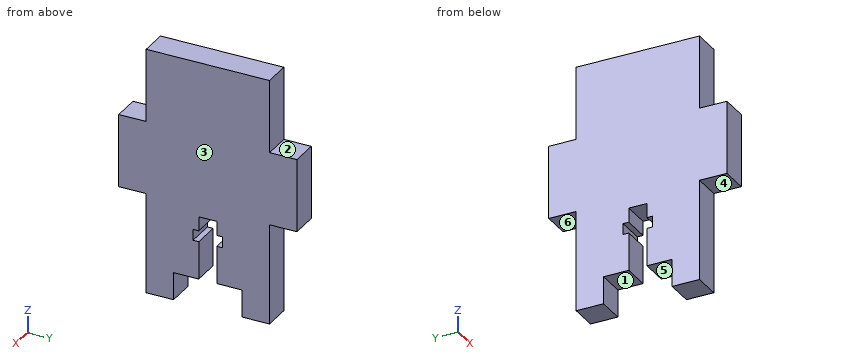
from build123d import *

# Parameters (mm, degrees)
SKETCH1_W           = 6.35
SKETCH1_H           = 28.575
BOSS_EXTRUDE1_DEPTH = 50.8
BOSS_EXTRUDE2_START = -34.925
SKETCH2_W           = 6.35
SKETCH2_H           = 16.933333334
BOSS_EXTRUDE2_DEPTH = 41.275
SKETCH3_W           = 6.35
SKETCH3_H           = 6.35
BOSS_EXTRUDE3_DEPTH = 6.35
CUT_EXTRUDE1_DEPTH  = 56.198450216


with BuildPart() as part:
    # Sketch1 → Boss-Extrude1 (new body)
    with BuildSketch(Plane.XY):
        with Locations((-25.4, 0)):
            Rectangle(SKETCH1_W, SKETCH1_H)
    extrude(amount=BOSS_EXTRUDE1_DEPTH)

    # Sketch2 → Boss-Extrude2 (add)
    with BuildSketch(Plane(origin=(0, -14.2875, 0), x_dir=(-1, 0, 0), z_dir=(0, -1, 0)).offset(BOSS_EXTRUDE2_START)):
        with Locations((25.4, -25.4)):
            Rectangle(SKETCH2_W, SKETCH2_H)
    extrude(amount=BOSS_EXTRUDE2_DEPTH)

    # Sketch3 → Boss-Extrude3 (add)
    with BuildSketch(Plane(origin=(0, 0, 0), x_dir=(-1, 0, 0), z_dir=(0, 0, -1))):
        with Locations((25.4, 11.1125)):
            Rectangle(SKETCH3_W, SKETCH3_H)
        with Locations((25.4, -11.1125)):
            Rectangle(SKETCH3_W, SKETCH3_H)
    extrude(amount=BOSS_EXTRUDE3_DEPTH)

    # Sketch4 → Cut-Extrude1 (cut, through all)
    with BuildSketch(Plane.ZY.offset(28.575)):
        Polygon((0, 2.0955), (0, -2.0955), (8.763, -2.0955), (8.763, -3.429), (11.303, -3.429), (11.303, -2.0955), (14.605, -2.0955), (14.605, 2.0955), (11.303, 2.0955), (11.303, 3.429), (8.763, 3.429), (8.763, 2.0955), align=None)
    extrude(amount=-CUT_EXTRUDE1_DEPTH, mode=Mode.SUBTRACT)


solid = part.part
The model under review builds one solid part; all positions refer to its coordinate system, in mm. Face numbers are marked on the shaded views. A direction names the side the tool comes from. Give positions to 0.01 mm unless a question says otherwise; leave off trailing zeros. Order: outer loops, then holes, each group sorted by start corner. A loop starts at its lowest first (then second) coordinate and runs counter-clockwise, first axis right, second up. Notation, with made-up numbers: M 80.25,48.5 L 114.25,48.5 A17 ccw 114.25,60.5 Z; hole C 31,19 d10. An arc over 180 degrees is marked long. Use one line per item in the form item = value. Start each with the question number.
Item 1: We need section C-C on y = 15.5. Give the boundary of the cut face in (x, z) (3 decimals).
Item 2: To check wall thickness, follow line 1 along Y through (x, z) = (-22.75, -3); line 2 along Y through (x, z) = (-26.5, 13); line 3 along Z through (x, y) = (-22.75, -2.5). State the ranges of each line that lie inside material, in increasing order. Write a range as from..to.
Item 3: The part is to be moulded in two halves that separate along Y. For the marked faces 5 and 6, say which applies: pulls with the +Y half, pulls with the -Y half, needs draft (parallel to the pull), parting line crosses it, or undercut.
Item 4: For the marked faces 1, 2, 3 and 4, list the 3-axis set-ups (+Z, -Z, +X, -X, +Y, -Y) from which the entire face can be reached by the end or side of a thin tool; tool diameter is ignored.
Item 5: We need section D-D on z = -1.5. Give the boundary of the cut face in (x, y) (1 decimal), plus the area to 3 significant figures.
Item 6: We need section A-A on z = 7. Give the boundary of the cut face in (x, y) (1 decimal).
Item 7: Insertion check: pin 1 Ø0.7 at (x, y) = (-24, -3) entering from -Z; pin 2 Ø3 at (x, y) = (-27.5, -16) entering from +Z; pin 3 Ø1.9 at (x, z) = (-25.5, 0) entering from +Y. Each pin has a flat end and moves straight along its axis. Give the tip position at first contact, or say it passes through.
Completed:
q1.outline = M -28.575,16.933 L -22.225,16.933 L -22.225,33.867 L -28.575,33.867 Z
q2.line_1 = -14.29..-7.94, 7.94..14.29
q2.line_2 = -14.29..-2.1, 2.1..14.29
q2.line_3 = 0..8.76, 11.3..50.8
q3.face_5 = undercut
q3.face_6 = needs draft
q4.face_1 = -Z, +X, -X
q4.face_2 = +Z, +X, -X, +Y
q4.face_3 = +Z, -Z, +X, +Y, -Y
q4.face_4 = -Z, +X, -X, -Y
q5.outline = M -28.6,-14.3 L -22.2,-14.3 L -22.2,-7.9 L -28.6,-7.9 Z; M -28.6,7.9 L -22.2,7.9 L -22.2,14.3 L -28.6,14.3 Z
q5.area = 80.6 mm²
q6.outline = M -28.6,-14.3 L -22.2,-14.3 L -22.2,-2.1 L -28.6,-2.1 Z; M -28.6,2.1 L -22.2,2.1 L -22.2,14.3 L -28.6,14.3 Z
q7.pin_1 = 0
q7.pin_2 = 33.87
q7.pin_3 = 14.29
